```python
from build123d import *

# Parameters (mm, degrees)
F1_DEPTH = 35
F3_DEPTH = 35.001
F4_R     = 1.5
F5_R     = 1.5


with BuildPart() as f1:
    # F0 (on Front) → F1 (new body)
    with BuildSketch(Plane.XZ):
        Polygon((26.035348, 24.228908), (-25.923712, 0), (31.076288, 0), (31.076288, 26.579537), align=None)
    extrude(amount=F1_DEPTH)

    # F2 (on face) → F3 (cut, through all)
    with BuildSketch(Plane.XZ.offset(35)):
        with BuildLine():
            Line((6.252536, 12.631768), (-7.342081, 6.292494))
            ThreePointArc((-7.342081, 6.292494), (-8.117693, 5.446063), (-8.067615, 4.299105))
            Line((-8.067615, 4.299105), (-7.644997, 3.392798))
            ThreePointArc((-7.644997, 3.392798), (-6.798566, 2.617186), (-5.651608, 2.667263))
            Line((-5.651608, 2.667263), (7.943009, 9.006537))
            ThreePointArc((7.943009, 9.006537), (8.71862, 9.852969), (8.668543, 10.999926))
            Line((8.668543, 10.999926), (8.245925, 11.906234))
            ThreePointArc((8.245925, 11.906234), (7.399493, 12.681846), (6.252536, 12.631768))
        make_face()
    extrude(amount=-F3_DEPTH, mode=Mode.SUBTRACT)

    # F4
    f4_edges = [f1.edges().sort_by_distance(p)[0] for p in [
        (-25.923712, -17.5, 0),
        (31.076288, -17.5, 26.579537),
    ]]
    fillet(f4_edges, radius=F4_R)

    # F5
    f5_edges = [f1.edges().sort_by_distance(p)[0] for p in [
        (31.076288, -35, 12.112504),
        (31.076288, 0, 12.112504),
    ]]
    fillet(f5_edges, radius=F5_R)


solid = f1.part
```
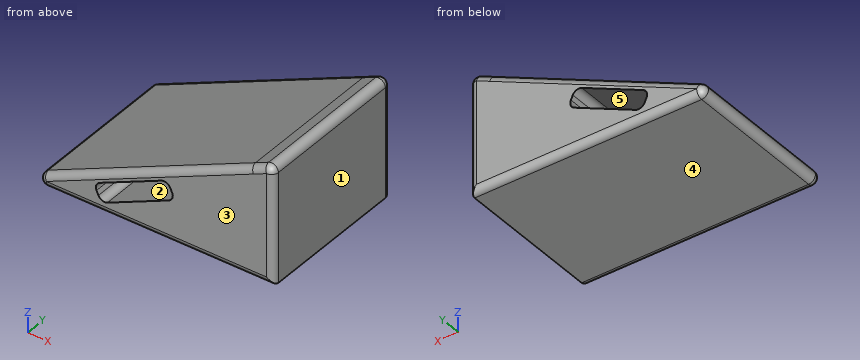
Check sheet for the modelled part. Datum: model origin and axes. Units: mm. Face numbers are marked on the shaded views. A direction names the side the tool comes from. Give positions to 0.01 mm unless a question says otherwise; leave off trailing zeros. Loops run counter-clockwise (first coordinate to the right, second up) from the corner with the lowest first, then second, coordinate; pieces in that order, holes last. Notation, with made-up numbers: M -9.5,-26.5 L 33.5,-26.5 A33 cw 33.5,6.5 Z; hole C 47,35 d10. An arc over 180 degrees is marked long. Answer in a Markdown table with one row per item.
1) Tool access check on the marked faces 1 and 2. Record the directions out of +Z, -Z, +X, -X, +Y, -Y that give a thin tool (end or side, any length) a straight path to the whole face; none if there is none.
Solutions:
| item | result |
|---|---|
| face 1 | +Z, -Z, +X, +Y, -Y |
| face 2 | +Y, -Y |
2) Depth check by flat-ended pin: pin 1 (12 mm diameter, centred on x = 16.5, y = -4, fed in from +Z); pin 2 (8 mm diameter, centred on y = -22, z = 9, fed in from -X); pin 3 (4 mm diameter, centred on x = 25.5, y = -30.5, fed in from +Z). Enter the tip coordinate at first touch or a pass-through.
Solutions:
| item | result |
|---|---|
| pin 1 | stops at z = 22.58 |
| pin 2 | stops at x = -15.2 |
| pin 3 | stops at z = 24.91 |
3) Cross-section at A-A (y = -15). Enter the section's corners in (x, z) (1 decimal).
Solutions:
| item | result |
|---|---|
| outline | M -19.8,2.9 A1.5 ccw -19.2,0 L 31.1,0 L 31.1,24.2 A1.5 ccw 28.9,25.6 Z; hole M -8.1,4.3 L -7.6,3.4 A1.5 ccw -5.7,2.7 L 7.9,9 A1.5 ccw 8.7,11 L 8.2,11.9 A1.5 ccw 6.3,12.6 L -7.3,6.3 A1.5 ccw Z |
4) Thickness scan on line 1 (Z direction, x = -12.5, y = -32); line 2 (Z direction, x = 6, y = -20); line 3 (X direction, y = -10.5, z = 10.75). Record the ranges inside material, lowest first.
Solutions:
| item | result |
|---|---|
| line 1 | z = 0 to 6.26 |
| line 2 | z = 0 to 8.1, 12.51 to 14.89 |
| line 3 | x = -2.87 to 2.22, 8.76 to 31.08 |
5) Mould release check, pull along Z, two halves, no side actions. Record for the marked faces 3, 4 and 5: released by +Z, released by -Z, zero draft, split by the parting line, or undercut.
Solutions:
| item | result |
|---|---|
| face 3 | zero draft |
| face 4 | released by -Z |
| face 5 | undercut |
